Input: part model. Units: mm. Frame: model coordinates. Face numbers are marked on the shaded views. A direction names the side the tool comes from. Give positions to 0.01 mm unless a question says otherwise; leave off trailing zeros. Order: outer loops, then holes, each group sorted by start corner. A loop starts at its lowest first (then second) coordinate and runs counter-clockwise, first axis right, second up. Notation, with made-up numbers: (76, 42.5) - (133, 42.5) arc R14 cw to (133, 46.5) - close; hole circle Ø9 at (88, -21.5). An arc over 180 degrees is marked (long way). Use a Markdown table: item, result.
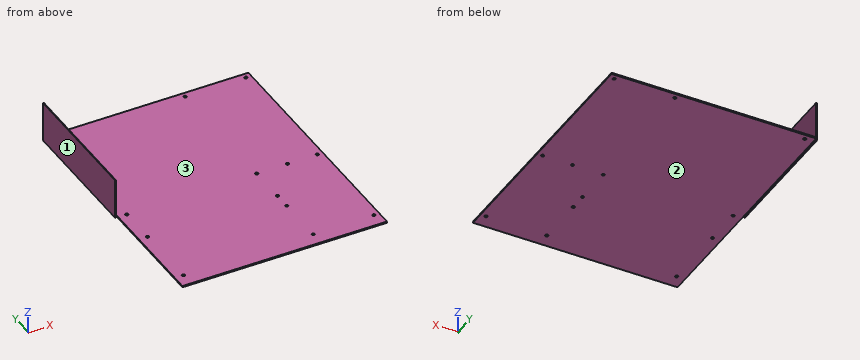
from build123d import *

# Parameters (mm, degrees)
SKETCH_1_W           = 244
SKETCH_1_H           = 305
EXTRUDE_1_DEPTH      = 1.6
SKETCH_2_R           = 1.75
CUT_EXTRUDE_1_DEPTH  = 391.593855558
EXTRUDE_2_DEPTH      = 44.45
EXTRUDE_2_DEPTH_BACK = 3.81
SKETCH_3_W           = 1
SKETCH_3_H           = 158.75


with BuildPart() as part:
    # 草图1 → 凸台-拉伸1 (new body)
    with BuildSketch(Plane.XY):
        with Locations((122, 152.5)):
            Rectangle(SKETCH_1_W, SKETCH_1_H)
    extrude(amount=EXTRUDE_1_DEPTH)

    # 草图2 → 切除-拉伸1 (cut, through all)
    with BuildSketch(Plane.XY.offset(1.6)):
        with Locations((10.16, 16.69)):
            Circle(SKETCH_2_R)
        with Locations((165.1, 16.69)):
            Circle(SKETCH_2_R)
        with Locations((237.49, 16.69)):
            Circle(SKETCH_2_R)
        with Locations((165.1, 75.11)):
            Circle(SKETCH_2_R)
        with Locations((10.16, 95.43)):
            Circle(SKETCH_2_R)
        with Locations((165.1, 95.43)):
            Circle(SKETCH_2_R)
        with Locations((10.16, 141.15)):
            Circle(SKETCH_2_R)
        with Locations((165.1, 141.15)):
            Circle(SKETCH_2_R)
        with Locations((237.49, 141.15)):
            Circle(SKETCH_2_R)
        with Locations((10.16, 298.63)):
            Circle(SKETCH_2_R)
        with Locations((165.1, 298.63)):
            Circle(SKETCH_2_R)
        with Locations((237.49, 298.63)):
            Circle(SKETCH_2_R)
        with Locations((201.816, 141.15)):
            Circle(SKETCH_2_R)
    extrude(amount=-CUT_EXTRUDE_1_DEPTH, mode=Mode.SUBTRACT)

    # 草图3 → 凸台-拉伸2 (add, two sides: drawn at the far end of the back side and taken through both)
    with BuildSketch(Plane.XY.offset(1.6).offset(-EXTRUDE_2_DEPTH_BACK)):
        with Locations((-0.5, 225.625)):
            Rectangle(SKETCH_3_W, SKETCH_3_H)
    extrude(amount=EXTRUDE_2_DEPTH + EXTRUDE_2_DEPTH_BACK)


solid = part.part
1. Pin query (flat end, axial travel): pin 1 (2 mm diameter, centred on x = 205, y = 157, fed in from +Z); pin 2 (0.5 mm diameter, centred on x = -0.5, z = 18, fed in from -Y); pin 3 (3 mm diameter, centred on x = 237.49, y = 298.63, fed in from +Z); pin 4 (8 mm diameter, centred on x = 109, y = 150.5, fed in from -Z). Return the tip coordinate at first contact, or that it passes through.
Response:
| item | result |
|---|---|
| pin 1 | stops at z = 1.6 |
| pin 2 | stops at y = 146.25 |
| pin 3 | passes through |
| pin 4 | stops at z = 0 |
2. Section query A-A (y = 210.5). Return loops of the section in (x, z).
Response:
| item | result |
|---|---|
| outline | (-1, -2.21) - (0, -2.21) - (0, 0) - (244, 0) - (244, 1.6) - (0, 1.6) - (0, 46.05) - (-1, 46.05) - close |
3. Section query B-B (z = 14). Return loops of the section in (x, y).
Response:
| item | result |
|---|---|
| outline | (-1, 146.25) - (0, 146.25) - (0, 305) - (-1, 305) - close |
4. Section query C-C (x = 105). Return loops of the section in (y, z), then the cut area to 3 significant figures.
Response:
| item | result |
|---|---|
| outline | (0, 0) - (305, 0) - (305, 1.6) - (0, 1.6) - close |
| area | 488 mm^2 |
5. Material intervals for line 1 along X through (y, z) = (141.15, 0.5); line 2 along Y through (x, z) = (165.1, 1.1); line 3 along X through (y, z) = (95.43, 0.9), sorted ascending.
Response:
| item | result |
|---|---|
| line 1 | x = 0 to 8.41, 11.91 to 163.35, 166.85 to 200.07, 203.57 to 235.74, 239.24 to 244 |
| line 2 | y = 0 to 14.94, 18.44 to 73.36, 76.86 to 93.68, 97.18 to 139.4, 142.9 to 296.88, 300.38 to 305 |
| line 3 | x = 0 to 8.41, 11.91 to 163.35, 166.85 to 244 |
6. Set-up query: the marked faces 1, 2 and 3. Return all of +Z, -Z, +X, -X, +Y, -Y with unobstructed straight access to the full face (end or side cutting, diameter ignored); none if empty.
Response:
| item | result |
|---|---|
| face 1 | +Z, -Z, -X, +Y, -Y |
| face 2 | -Z, +X, +Y, -Y |
| face 3 | +Z, +X, +Y, -Y |
